```python
from build123d import *

# Parameters (mm, degrees)
EXTRUDE_1_DEPTH          = 10
SKETCH_2_R               = 2.752434458
CUT_EXTRUDE_1_DEPTH      = 1
CUT_EXTRUDE_1_DEPTH_BACK = 11


with BuildPart() as part:
    # 草图1 → 凸台-拉伸1 (new body)
    with BuildSketch(Plane(origin=(0, 0, 0), x_dir=(1, 0, 0), z_dir=(0, 1, 0))):
        with BuildLine():
            ThreePointArc((1.117051771, 21.971622501), (-0.045961741, 19.869637729), (-0.410530178, 17.495184051))
            ThreePointArc((-0.410530178, 17.495184051), (-1.373034175, 17.44605334), (-2.331373887, 17.344010372))
            ThreePointArc((-2.331373887, 17.344010372), (-3.062900273, 19.632199517), (-4.540418022, 21.526369972))
            ThreePointArc((-4.540418022, 21.526369972), (-5.135798005, 21.392138249), (-5.727225381, 21.241442734))
            ThreePointArc((-5.727225381, 21.241442734), (-6.183767943, 18.882945479), (-5.796746593, 16.512047994))
            ThreePointArc((-5.796746593, 16.512047994), (-6.696960066, 16.167891819), (-7.576862283, 15.774699932))
            ThreePointArc((-7.576862283, 15.774699932), (-8.979674551, 17.724843043), (-10.970208295, 19.069728104))
            ThreePointArc((-10.970208295, 19.069728104), (-11.494968424, 18.758083616), (-12.010881809, 18.432002554))
            ThreePointArc((-12.010881809, 18.432002554), (-11.716263855, 16.047858961), (-10.615537062, 13.912597632))
            ThreePointArc((-10.615537062, 13.912597632), (-11.365340846, 13.307104398), (-12.080674608, 12.661251953))
            ThreePointArc((-12.080674608, 12.661251953), (-14.017455719, 14.082455436), (-16.326158146, 14.746408382))
            ThreePointArc((-16.326158146, 14.746408382), (-16.728931243, 14.287857063), (-17.118829441, 13.818309541))
            ThreePointArc((-17.118829441, 13.818309541), (-16.101890228, 11.641896196), (-14.395204801, 9.95128528))
            ThreePointArc((-14.395204801, 9.95128528), (-14.921202876, 9.143724883), (-15.40194633, 8.308432417))
            ThreePointArc((-15.40194633, 8.308432417), (-17.683110656, 9.061578973), (-20.083989887, 8.979607464))
            ThreePointArc((-20.083989887, 8.979607464), (-20.325349715, 8.419035512), (-20.551066773, 7.851984112))
            ThreePointArc((-20.551066773, 7.851984112), (-18.911351397, 6.096343517), (-16.765769597, 5.01587179))
            ThreePointArc((-16.765769597, 5.01587179), (-17.016473607, 4.085293867), (-17.215568235, 3.142325628))
            ThreePointArc((-17.215568235, 3.142325628), (-19.617819516, 3.153692024), (-21.875860765, 2.333820002))
            ThreePointArc((-21.875860765, 2.333820002), (-21.932181342, 1.726100106), (-21.971622501, 1.117051771))
            ThreePointArc((-21.971622501, 1.117051771), (-19.869637729, -0.045961741), (-17.495184051, -0.410530178))
            ThreePointArc((-17.495184051, -0.410530178), (-17.44605334, -1.373034175), (-17.344010372, -2.331373887))
            ThreePointArc((-17.344010372, -2.331373887), (-19.632199517, -3.062900273), (-21.526369972, -4.540418022))
            ThreePointArc((-21.526369972, -4.540418022), (-21.392138249, -5.135798005), (-21.241442734, -5.727225381))
            ThreePointArc((-21.241442734, -5.727225381), (-18.882945479, -6.183767943), (-16.512047994, -5.796746593))
            ThreePointArc((-16.512047994, -5.796746593), (-16.167891819, -6.696960066), (-15.774699932, -7.576862283))
            ThreePointArc((-15.774699932, -7.576862283), (-17.724843043, -8.979674551), (-19.069728104, -10.970208295))
            ThreePointArc((-19.069728104, -10.970208295), (-18.758083616, -11.494968424), (-18.432002554, -12.010881809))
            ThreePointArc((-18.432002554, -12.010881809), (-16.047858961, -11.716263855), (-13.912597632, -10.615537062))
            ThreePointArc((-13.912597632, -10.615537062), (-13.307104398, -11.365340846), (-12.661251953, -12.080674608))
            ThreePointArc((-12.661251953, -12.080674608), (-14.082455436, -14.017455719), (-14.746408382, -16.326158146))
            ThreePointArc((-14.746408382, -16.326158146), (-14.287857063, -16.728931243), (-13.818309541, -17.118829441))
            ThreePointArc((-13.818309541, -17.118829441), (-11.641896196, -16.101890228), (-9.95128528, -14.395204801))
            ThreePointArc((-9.95128528, -14.395204801), (-9.143724883, -14.921202876), (-8.308432417, -15.40194633))
            ThreePointArc((-8.308432417, -15.40194633), (-9.061578973, -17.683110656), (-8.979607464, -20.083989887))
            ThreePointArc((-8.979607464, -20.083989887), (-8.419035512, -20.325349715), (-7.851984112, -20.551066773))
            ThreePointArc((-7.851984112, -20.551066773), (-6.096343517, -18.911351397), (-5.01587179, -16.765769597))
            ThreePointArc((-5.01587179, -16.765769597), (-4.085293867, -17.016473607), (-3.142325628, -17.215568235))
            ThreePointArc((-3.142325628, -17.215568235), (-3.153692024, -19.617819516), (-2.333820002, -21.875860765))
            ThreePointArc((-2.333820002, -21.875860765), (-1.726100106, -21.932181342), (-1.117051771, -21.971622501))
            ThreePointArc((-1.117051771, -21.971622501), (0.045961741, -19.869637729), (0.410530178, -17.495184051))
            ThreePointArc((0.410530178, -17.495184051), (1.373034175, -17.44605334), (2.331373887, -17.344010372))
            ThreePointArc((2.331373887, -17.344010372), (3.062900273, -19.632199517), (4.540418022, -21.526369972))
            ThreePointArc((4.540418022, -21.526369972), (5.135798005, -21.392138249), (5.727225381, -21.241442734))
            ThreePointArc((5.727225381, -21.241442734), (6.183767943, -18.882945479), (5.796746593, -16.512047994))
            ThreePointArc((5.796746593, -16.512047994), (6.696960066, -16.167891819), (7.576862283, -15.774699932))
            ThreePointArc((7.576862283, -15.774699932), (8.979674551, -17.724843043), (10.970208295, -19.069728104))
            ThreePointArc((10.970208295, -19.069728104), (11.494968424, -18.758083616), (12.010881809, -18.432002554))
            ThreePointArc((12.010881809, -18.432002554), (11.716263855, -16.047858961), (10.615537062, -13.912597632))
            ThreePointArc((10.615537062, -13.912597632), (11.365340846, -13.307104398), (12.080674608, -12.661251953))
            ThreePointArc((12.080674608, -12.661251953), (14.017455719, -14.082455436), (16.326158146, -14.746408382))
            ThreePointArc((16.326158146, -14.746408382), (16.728931243, -14.287857063), (17.118829441, -13.818309541))
            ThreePointArc((17.118829441, -13.818309541), (16.101890228, -11.641896196), (14.395204801, -9.95128528))
            ThreePointArc((14.395204801, -9.95128528), (14.921202876, -9.143724883), (15.40194633, -8.308432417))
            ThreePointArc((15.40194633, -8.308432417), (17.683110656, -9.061578973), (20.083989887, -8.979607464))
            ThreePointArc((20.083989887, -8.979607464), (20.325349715, -8.419035512), (20.551066773, -7.851984112))
            ThreePointArc((20.551066773, -7.851984112), (18.911351397, -6.096343517), (16.765769597, -5.01587179))
            ThreePointArc((16.765769597, -5.01587179), (17.016473607, -4.085293867), (17.215568235, -3.142325628))
            ThreePointArc((17.215568235, -3.142325628), (19.617819516, -3.153692024), (21.875860765, -2.333820002))
            ThreePointArc((21.875860765, -2.333820002), (21.932181342, -1.726100106), (21.971622501, -1.117051771))
            ThreePointArc((21.971622501, -1.117051771), (19.869637729, 0.045961741), (17.495184051, 0.410530178))
            ThreePointArc((17.495184051, 0.410530178), (17.44605334, 1.373034175), (17.344010372, 2.331373887))
            ThreePointArc((17.344010372, 2.331373887), (19.632199517, 3.062900273), (21.526369972, 4.540418022))
            ThreePointArc((21.526369972, 4.540418022), (21.392138249, 5.135798005), (21.241442734, 5.727225381))
            ThreePointArc((21.241442734, 5.727225381), (18.882945479, 6.183767943), (16.512047994, 5.796746593))
            ThreePointArc((16.512047994, 5.796746593), (16.167891819, 6.696960066), (15.774699932, 7.576862283))
            ThreePointArc((15.774699932, 7.576862283), (17.724843043, 8.979674551), (19.069728104, 10.970208295))
            ThreePointArc((19.069728104, 10.970208295), (18.758083616, 11.494968424), (18.432002554, 12.010881809))
            ThreePointArc((18.432002554, 12.010881809), (16.047858961, 11.716263855), (13.912597632, 10.615537062))
            ThreePointArc((13.912597632, 10.615537062), (13.307104398, 11.365340846), (12.661251953, 12.080674608))
            ThreePointArc((12.661251953, 12.080674608), (14.082455436, 14.017455719), (14.746408382, 16.326158146))
            ThreePointArc((14.746408382, 16.326158146), (14.287857063, 16.728931243), (13.818309541, 17.118829441))
            ThreePointArc((13.818309541, 17.118829441), (11.641896196, 16.101890228), (9.95128528, 14.395204801))
            ThreePointArc((9.95128528, 14.395204801), (9.143724883, 14.921202876), (8.308432417, 15.40194633))
            ThreePointArc((8.308432417, 15.40194633), (9.061578973, 17.683110656), (8.979607464, 20.083989887))
            ThreePointArc((8.979607464, 20.083989887), (8.419035512, 20.325349715), (7.851984112, 20.551066773))
            ThreePointArc((7.851984112, 20.551066773), (6.096343517, 18.911351397), (5.01587179, 16.765769597))
            ThreePointArc((5.01587179, 16.765769597), (4.085293867, 17.016473607), (3.142325628, 17.215568235))
            ThreePointArc((3.142325628, 17.215568235), (3.153692024, 19.617819516), (2.333820002, 21.875860765))
            ThreePointArc((2.333820002, 21.875860765), (1.726100106, 21.932181342), (1.117051771, 21.971622501))
        make_face()
    extrude(amount=EXTRUDE_1_DEPTH)

    # 草图2 → 切除-拉伸1 (cut, two sides)
    with BuildSketch(Plane(origin=(0, 10, 0), x_dir=(1, 0, 0), z_dir=(0, 1, 0))) as cut_extrude_1_sk:
        Circle(SKETCH_2_R)
    extrude(amount=CUT_EXTRUDE_1_DEPTH, mode=Mode.SUBTRACT)
    extrude(cut_extrude_1_sk.sketch, amount=-CUT_EXTRUDE_1_DEPTH_BACK, mode=Mode.SUBTRACT)


solid = part.part
```
Source: CAD feature listing. Evaluate the final solid. Frame: model axes, mm. A direction names the side the tool comes from. Coordinates: 2 decimals unless noted, no trailing zeros. Answer as a JSON object with one key per item and string values.
1. Draft query along X for faces 5 (the cylindrical face through (-1.73, 4.93, 21.93)), 6 (the cylindrical face through (-6.684, 4.93, -16.173)), 7 (the cylindrical face through (16.12, 4.93, 11.67)), 8 (the cylindrical face through (2.625, 5.07, -0.827)). Return one class per face: released by +X, released by -X, zero draft, split by the parting line, or undercut.
Evaluation:
{"face 5": "released by -X", "face 6": "undercut", "face 7": "released by +X", "face 8": "undercut"}
2. Access query for faces 1 (the cylindrical face through (17.447, 4.93, -1.36)), 2 (the cylindrical face through (13.316, 4.93, -11.355)), 3 (the cylindrical face through (-16.12, 4.93, -11.67)), 4 (the cylindrical face through (11.67, 4.93, -16.12)). Directions: +Z, -Z, +X, -X, +Y, -Y. A direction counts if a zero-diameter tool reaches every point of the face in a straight line with its end or side. Return the directions, or none.
Evaluation:
{"face 1": "+X, +Y, -Y", "face 2": "+Y, -Y", "face 3": "-X, +Y, -Y", "face 4": "-Z, +Y, -Y"}
3. Ray query, L1, parallel to Z at x = -15.5, y = 4.5; L2, parallel to X at y = 7, z = -13; L3, parallel to X at y = 6.5, z = -12.5. Return the intervals inside material, ascending.
Evaluation:
{"L1": "-14.61 to -10.9, -8.36 to 11.52", "L2": "-16.84 to -12.43, -11.72 to 13.47", "L3": "-16.62 to 13.07"}
4. Contact query for flat-ended pins moving along their axis: P1, Ø2, axis at y = 3, z = -11.5, coming from the -X side; P2, Ø1.5, axis at x = -2, y = 4.5, coming from the +Z side; P3, Ø2, axis at y = 4, z = -10, coming from the +X side; P4, Ø5, axis at x = 0, z = 0, coming from the +Y side. Output: stop coordinate, or through.
Evaluation:
{"P1": "x = -16.62", "P2": "z = 21.96", "P3": "x = 19.07", "P4": "through"}
